Design review of the part shown in the three views and the two pictorial views. Dimensions are in mm from the part's minimum x, y and z. A direction names the side the tool comes from. Round coordinates to 2 decimals unless told otherwise and drop trailing zeros. Loops run counter-clockwise (first coordinate to the right, second up) from the corner with the lowest first, then second, coordinate; pieces in that order, holes last. Notation, with made-up numbers: (85, 65) -> (102, 65) arc R25 ccw to (102, 91) -> close; hole circle Ø7 at (78, 69). An arc over 180 degrees is marked (long way). Use a Markdown table: item, result. Add a question column.
1) Consider section C-C on x = 7.5. Give the boundary of the cut face in (y, z), plus the area to 3 significant figures.
2) For the marked faces 1 and 2, list the 3-axis set-ups (+Z, -Z, +X, -X, +Y, -Y) from which the entire face can be reached by the end or side of a thin tool; tool diameter is ignored.
3) Consider section A-A on y = 55. Give the boundary of the cut face in (x, z).
4) Insertion check: pin 1 (5.5 mm diameter, centred on y = 145, z = 25, fed in from +X); pin 2 (1 mm diameter, centred on y = 160.5, z = 40.5, fed in from +X); pin 3 (8 mm diameter, centred on x = 25, z = 25, fed in from -Y). Each pin has a flat end and moves straight along its axis. Give the tip position at first contact, or say it passes through.
5) Wall thickness on probe 1 along Y at (x, z) = (2.15, 25); probe 2 along Z at (x, y) = (2, 145); probe 3 along Y at (x, z) = (21.5, 40): over which ranges is each line inside the solid? List them lowest first.
6) Consider section D-D on z = 15. Give the boundary of the cut face in (x, y), plus the area to 3 significant figures.
7) Consider section B-B on x = 25. Give the boundary of the cut face in (y, z), plus the area to 3 significant figures.
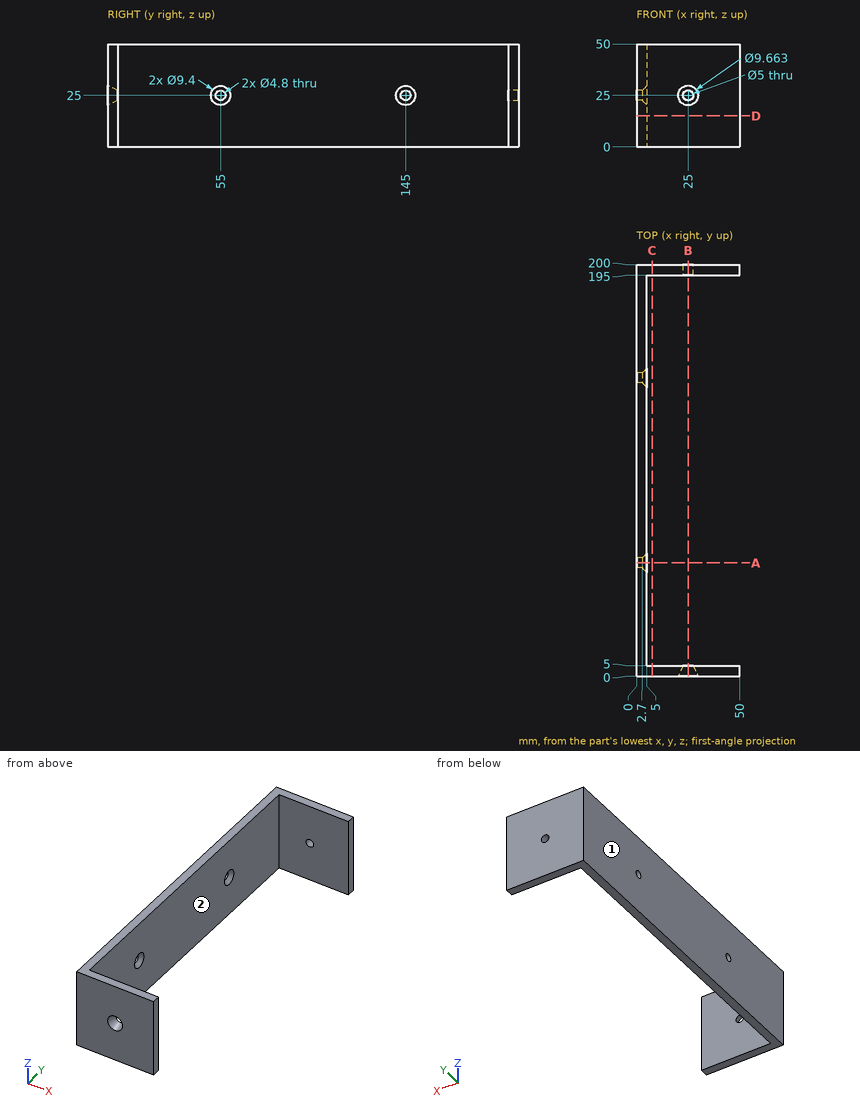
Result set:
| question | item | result |
|---|---|---|
| 1 | outline | (0, 0) -> (5, 0) -> (5, 50) -> (0, 50) -> close; (195, 0) -> (200, 0) -> (200, 50) -> (195, 50) -> close |
| 1 | area | 500 mm2 |
| 2 | face 1 | +Z, -Z, -X, +Y, -Y |
| 2 | face 2 | +Z, -Z, +X |
| 3 | outline | (0, 0) -> (5, 0) -> (5, 20.3) -> (2.7, 22.6) -> (0, 22.6) -> close; (0, 27.4) -> (2.7, 27.4) -> (5, 29.7) -> (5, 50) -> (0, 50) -> close |
| 4 | pin 1 | x = 3.05 |
| 4 | pin 2 | x = 5 |
| 4 | pin 3 | y = 1.78 |
| 5 | probe 1 | 0 to 52.6, 57.4 to 142.6, 147.4 to 200 |
| 5 | probe 2 | 0 to 22.6, 27.4 to 50 |
| 5 | probe 3 | 0 to 5, 195 to 200 |
| 6 | outline | (0, 0) -> (50, 0) -> (50, 5) -> (5, 5) -> (5, 195) -> (50, 195) -> (50, 200) -> (0, 200) -> close |
| 6 | area | 1,450 mm2 |
| 7 | outline | (0, 0) -> (5, 0) -> (5, 22.5) -> (0, 20.17) -> close; (0, 29.83) -> (5, 27.5) -> (5, 50) -> (0, 50) -> close; (195, 0) -> (200, 0) -> (200, 22.5) -> (195, 22.5) -> close; (195, 27.5) -> (200, 27.5) -> (200, 50) -> (195, 50) -> close |
| 7 | area | 438 mm2 |
